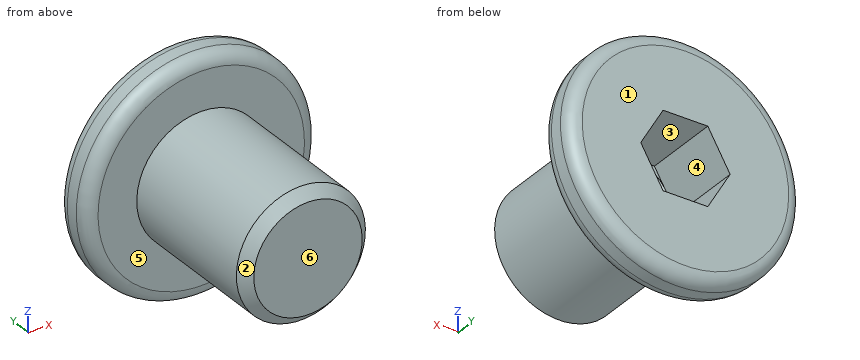
```python
from build123d import *

# Parameters (mm, degrees)
CUT_EXTRUDE2_DEPTH = 3


with BuildPart() as part:
    # Sketch1 → Revolve1 (revolve)
    with BuildSketch(Plane.XY, mode=Mode.PRIVATE) as revolve1_sk:
        with BuildLine():
            Line((-4.5, -0.5), (-4.5, -1))
            ThreePointArc((-4.5, -1), (-4.353553391, -1.353553391), (-4, -1.5))
            Line((-4, -1.5), (-2.5, -1.5))
            Line((-2.5, -1.5), (-2.5, -7.1))
            Line((-2.5, -7.1), (-2.1, -7.5))
            Line((-2.1, -7.5), (0, -7.5))
            Line((0, -7.5), (0, -4))
            Line((0, -4), (-1.5, -3))
            Line((-1.5, -3), (-1.5, 0))
            Line((-1.5, 0), (-4, 0))
            ThreePointArc((-4, 0), (-4.353553391, -0.146446609), (-4.5, -0.5))
        make_face()
    revolve(revolve1_sk.sketch.rotate(Axis((0, 2.75, 0), (0, -1, 0)), 270), axis=Axis((0, 2.75, 0), (0, -1, 0)))

    # Sketch3 → Cut-Extrude2 (cut)
    with BuildSketch(Plane(origin=(0, 0, 0), x_dir=(1, 0, 0), z_dir=(0, 1, 0))):
        Polygon((-0.866025404, -1.5), (0.866025404, -1.5), (1.732050808, 0), (0.866025404, 1.5), (-0.866025404, 1.5), (-1.732050808, 0), align=None)
    extrude(amount=-CUT_EXTRUDE2_DEPTH, mode=Mode.SUBTRACT)


solid = part.part
```
Work out the finished part from the listing and answer in its coordinate system (mm). Face numbers are marked on the shaded views. A direction names the side the tool comes from. Round coordinates to 2 decimals unless told otherwise and drop trailing zeros. Write each loop counter-clockwise with the first axis right and the second up, starting at its lowest first coordinate (ties: lowest second). Pieces come first, ordered by that corner, then holes. Notation, with made-up numbers: (-35, -36) - (22, -36) arc R23 ccw to (22, -14) - close; hole circle Ø8 at (38.25, -12.5). An arc over 180 degrees is marked (long way). Return JSON: item names as keys, results as strings. Group by question number.
Q1. For the marked faces 4, 5 and 6, determine the directions among +Z, -Z, +X, -X, +Y, -Y from which every point of the face is accessible in a straight line to the end or side of a thin tool.
Q2. The mould has two halves that part along Z. Classify the marked faces 1, 2 and 3: released by +Z, released by -Z, zero draft, split by the parting line, or undercut.
Q3. Each of these flat-tipped pins is pushed along its axis until it touches: pin 1 Ø4 at (x, y) = (2.5, -3) entering from -Z; pin 2 Ø0.5 at (x, y) = (-0.5, -1.5) entering from +Z; pin 3 Ø0.9 at (x, y) = (0.5, -1.5) entering from -Z. Where does it stop, or does it pass through?
Q4. Find the intervals of material crossed by L1, parallel to Z at x = 0.5, y = -0.5; L2, parallel to Y at x = -3.5, z = -0.5; L3, parallel to Z at x = 1.5, y = -2.5, in increasing order.
Q5. The part is cut by section A-A on y = -5. Write down the section's boundary in (x, z).
Q6. The part is cut by section B-B on y = -3.25. Write down the section's boundary in (x, z) (3 decimals), then the cut area to 3 significant figures.
Solved:
{
 "1": {"face 4": "+Y", "face 5": "-Y", "face 6": "+Z, -Z, +X, -X, -Y"},
 "2": {"face 1": "zero draft", "face 2": "split by the parting line", "face 3": "undercut"},
 "3": {"pin 1": "z = -4.16", "pin 2": "z = 4.41", "pin 3": "z = -4.48"},
 "4": {"L1": "-4.47 to -1.5, 1.5 to 4.47", "L2": "-1.5 to 0", "L3": "-2 to -0.4, 0.4 to 2"},
 "5": {"outline": "circle Ø5 at (0, 0)"},
 "6": {"outline": "circle Ø5 at (0, 0); hole circle Ø2.25 at (0, 0)", "area": "15.7 mm²"}
}
